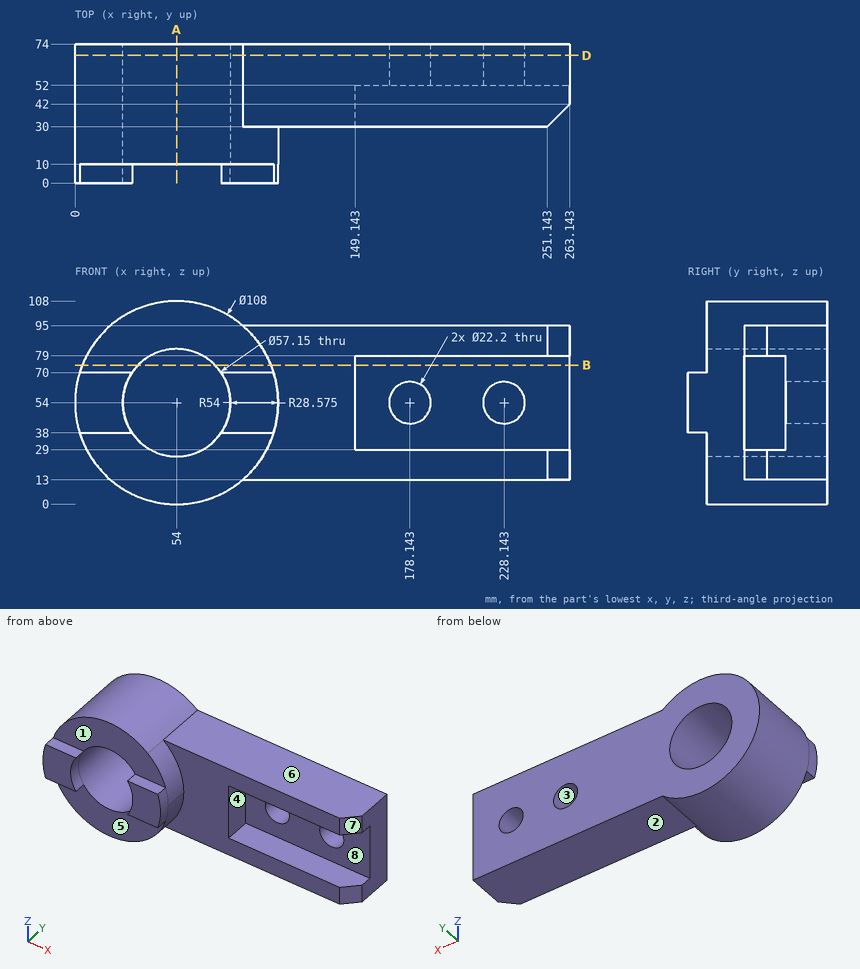
The drawing under review shows one solid part. Ordinate dimensions are in mm from its lowest x, y, z. A direction names the side the tool comes from. Round coordinates to 2 decimals unless told otherwise and drop trailing zeros. Order: outer loops, then holes, each group sorted by start corner. A loop starts at its lowest first (then second) coordinate and runs counter-clockwise, first axis right, second up. Notation, with made-up numbers: (73.25, 2) -> (110.25, 2) arc R22 ccw to (110.25, 8) -> close; hole circle Ø4 at (27.5, 18). An arc over 180 degrees is marked (long way). Use a Markdown table: item, result.
Item 1: Take a section at D-D (y = 68). State how many separate pieces and enclosed holes the cut face has, plus the area to 3 significant figures.
Resolved:
| item | result |
|---|---|
| separate pieces | 1 |
| enclosed holes | 3 |
| area | 19,000 mm² |
Item 2: Draft analysis for pull direction Z (two halves, no side actions). For the marked faces 6, 7 and 8, state which applies: +Z half, -Z half, draft (parallel to the pull), parting line (faces both ways), or undercut.
Resolved:
| item | result |
|---|---|
| face 6 | +Z half |
| face 7 | draft |
| face 8 | undercut |
Item 3: Take a section at A-A (x = 54). State the section outline as (y, z) points (1 decimal).
Resolved:
| item | result |
|---|---|
| outline | (10, 0) -> (74, 0) -> (74, 25.4) -> (10, 25.4) -> close; (10, 82.6) -> (74, 82.6) -> (74, 108) -> (10, 108) -> close |
Item 4: Machinability: for the marked faces 1, 2, 3, 4 and 5, which of the approach directions +Z, -Z, +X, -X, +Y, -Y give a long, thin tool a straight path to every point of the face, cutting with its end or side? Answer none if there is none.
Resolved:
| item | result |
|---|---|
| face 1 | +Z, +X, -X, -Y |
| face 2 | -Z, +X, +Y, -Y |
| face 3 | +Y, -Y |
| face 4 | +X, -Y |
| face 5 | -Z, +X, -X, -Y |
Item 5: For pin 1 (17.5 mm diameter, centred on y = 42, z = 43.5, fed in from +X); pin 2 (6 mm diameter, centred on x = 179.5, y = 57.5, fed in from -Z); pin 3 (1 mm diameter, centred on x = 177.5, z = 21, fed in from -Y); pin 4 (18 mm diameter, centred on x = 178.14, z = 54, fed in from -Y), all flat-tipped, find the tip position at first contact; note any pin that passes through.
Resolved:
| item | result |
|---|---|
| pin 1 | stops at x = 149.14 |
| pin 2 | stops at z = 13 |
| pin 3 | stops at y = 30 |
| pin 4 | passes through |
Item 6: Take a section at B-B (z = 74). State the section outline as (x, y) points.
Resolved:
| item | result |
|---|---|
| outline | (3.84, 10) -> (33.59, 10) -> (33.59, 74) -> (3.84, 74) -> close; (74.41, 10) -> (104.16, 10) -> (104.16, 30) -> (149.14, 30) -> (149.14, 52) -> (263.14, 52) -> (263.14, 74) -> (74.41, 74) -> close |
Item 7: For line 1 along X through (y, z) = (67.25, 54) (1 decimal); line 2 along Z through (x, y) = (187, 35.5); line 3 along Z through (x, y) = (54, 45.5) (1 decimal), list the stretches that pass through material, from the lowest coordinate up. Write a range as [from, to].
Resolved:
| item | result |
|---|---|
| line 1 | x = [0, 25.4], [82.6, 167], [189.2, 217], [239.2, 263.1] |
| line 2 | z = [13, 29], [79, 95] |
| line 3 | z = [0, 25.4], [82.6, 108] |
